Work out the finished part from the listing and answer in its coordinate system (mm). A direction names the side the tool comes from. Give positions to 0.01 mm unless a question says otherwise; leave off trailing zeros. Order: outer loops, then holes, each group sorted by start corner. A loop starts at its lowest first (then second) coordinate and runs counter-clockwise, first axis right, second up. Notation, with made-up numbers: (-33.75, 27.5) - (0.25, 27.5) arc R20 ccw to (0.25, 40.5) - close; hole circle Ø9 at (7.25, 32). An arc over 180 degrees is marked (long way). Put each result on its own line as item: value.
```python
from build123d import *

# Parameters (mm, degrees)
REVOLVE1_ANGLE      = 75
FILLET1_R           = 80
FILLET2_R           = 80
SKETCH3_W           = 220
SKETCH3_H           = 208.906104004
CUT_EXTRUDE3_DEPTH  = 159
BOSS_EXTRUDE1_START = -20
BOSS_EXTRUDE1_DEPTH = 20
SKETCH6_W           = 10
SKETCH6_H           = 10
CUT_EXTRUDE4_DEPTH  = 10


with BuildPart() as part:
    # Sketch1 → Revolve1 (revolve)
    with BuildSketch(Plane.XY):
        with BuildLine():
            Line((0, 0), (3.000014971, 0))
            Line((3.000014971, 0), (2.999985029, 0.009477573))
            add(Edge.make_bspline(
                [(2.999985029, 0.009477573), (2.993785153, 1.971956174), (2.98195041, 5.919056141), (3.145368661, 11.706950418), (3.673805689, 17.348455242), (4.826995442, 22.758009885), (6.767385374, 27.848912294), (10.462264152, 34.106073266), (16.932254921, 40.80886219), (26.377617743, 47.258644811), (36.67301066, 52.572311975), (47.441384771, 57.081049673), (62.17748954, 62.31037411), (81.042213455, 67.757539775), (104.018152235, 73.218909741), (126.982089983, 77.893970447), (142.347775171, 80.65244689), (149.958103424, 81.949720096), (150, 81.956859546)],
                knots=[0, 0, 0, 0, 0.03125, 0.0625, 0.09375, 0.125, 0.15625, 0.1875, 0.25, 0.3125, 0.375, 0.4375, 0.5, 0.625, 0.75, 0.875, 0.996633751, 0.997307001, 0.997307001, 0.997307001, 0.997307001], degree=3))
            Line((150, 81.956859546), (530, 81.956859546))
            Line((530, 81.956859546), (530, 85))
            Line((530, 85), (150, 85))
            add(Edge.make_bspline(
                [(0, 0), (-0.012294225, 3.891554312), (-0.027437579, 8.684958126), (0.361573767, 14.085722357), (0.576098453, 16.090496183), (0.782493435, 17.604822189), (0.986227589, 18.854298664), (1.188670863, 19.931536976), (1.390404268, 20.885679324), (1.591698837, 21.746529091), (1.792703864, 22.533746067), (1.993507167, 23.261083862), (2.253808552, 24.139979457), (2.580573656, 25.146175179), (2.983585386, 26.259501153), (3.385879093, 27.271261727), (3.787683439, 28.201566994), (4.189138614, 29.064817448), (4.590335615, 29.871726974), (5.05331092, 30.74778076), (5.583218589, 31.683457084), (6.185429632, 32.669732492), (6.787226927, 33.590624245), (7.451481511, 34.546094958), (8.182770444, 35.530963646), (8.985083876, 36.540013411), (9.850344603, 37.562485558), (10.782608842, 38.595746542), (11.785011743, 39.636928062), (12.851029789, 40.680352273), (13.983960321, 41.72463117), (15.186170623, 42.768194245), (16.387975322, 43.755294725), (17.654380903, 44.743506811), (18.987602276, 45.731471932), (20.389198856, 46.717890971), (21.790522044, 47.657861765), (23.257103599, 48.59836715), (24.790441056, 49.538186318), (26.391587757, 50.476245251), (28.05829275, 51.412163763), (29.791720393, 52.345056651), (31.59268286, 53.274185034), (33.459445798, 54.199628429), (35.392909821, 55.120726442), (37.459746918, 56.067201212), (39.59327023, 57.006562681), (41.860151348, 57.96659169), (44.193707143, 58.917521836), (46.660609333, 59.885320784), (49.260404933, 60.867669295), (51.99403381, 61.861671206), (54.860992187, 62.865616104), (57.794602823, 63.85555089), (60.861539281, 64.853573463), (64.06149587, 65.858380358), (67.461497598, 66.888166734), (70.995135905, 67.920234745), (74.662088876, 68.953918346), (78.462130407, 69.988575944), (82.462197069, 71.040436012), (86.662284614, 72.107100186), (91.062388571, 73.18640193), (95.662505252, 74.276388609), (100.462631288, 75.375305679), (105.462763855, 76.481579791), (110.662900527, 77.593803027), (116.063039296, 78.710717608), (121.663178505, 79.831201671), (127.529872228, 80.967142806), (133.663251007, 82.116215238), (140.063409966, 83.276352633), (145.198462089, 84.177415336), (148.333178957, 84.715838785), (149.39998937, 84.897876633), (149.733326587, 84.954653305), (149.933332963, 84.98866355), (150, 85)],
                knots=[0, 0, 0, 0, 0.061462209, 0.075705788, 0.085548437, 0.093321935, 0.099856333, 0.105553797, 0.110642995, 0.115267654, 0.119524592, 0.123482434, 0.127191759, 0.134010181, 0.140199136, 0.145901384, 0.151215493, 0.156212588, 0.160945789, 0.165455878, 0.171870938, 0.177937368, 0.183716425, 0.189254732, 0.196326298, 0.203099892, 0.209625632, 0.217492532, 0.225090541, 0.232464167, 0.24106462, 0.249438142, 0.257620809, 0.265641058, 0.274822876, 0.28384341, 0.292725747, 0.301488561, 0.311376345, 0.321146599, 0.330814589, 0.341584449, 0.352255608, 0.362840299, 0.374512001, 0.386101174, 0.398765505, 0.411352526, 0.425006218, 0.438588433, 0.453231339, 0.468927603, 0.484557057, 0.501237456, 0.517857889, 0.535527769, 0.554243231, 0.574001115, 0.593705628, 0.614453399, 0.636242373, 0.65907093, 0.682937829, 0.707842151, 0.733783254, 0.760760729, 0.78877436, 0.81782409, 0.847909993, 0.879032247, 0.912262482, 0.946527454, 0.981827786, 0.994656092, 0.99679374, 0.998931275, 1, 1, 1, 1], degree=3))
        make_face()
    revolve(axis=Axis((0, 0, 0), (1, 0, 0)), revolution_arc=REVOLVE1_ANGLE)

    # Fillet1
    fillet1_edges = [part.edges().sort_by_distance(p)[0] for p in [
        (150, 65.020748281, 49.892174934),
    ]]
    fillet(fillet1_edges, radius=FILLET1_R)

    # Fillet2
    fillet2_edges = [part.edges().sort_by_distance(p)[0] for p in [
        (150, 67.435033925, 51.744721466),
    ]]
    fillet(fillet2_edges, radius=FILLET2_R)

    # Sketch3 → Cut-Extrude3 (cut)
    with BuildSketch(Plane(origin=(0, 0, 0), x_dir=(1, 0, 0), z_dir=(0, 1, 0))):
        Rectangle(SKETCH3_W, SKETCH3_H)
    extrude(amount=CUT_EXTRUDE3_DEPTH, mode=Mode.SUBTRACT)

    # Sketch5 → Boss-Extrude1 (add)
    with BuildSketch(Plane(origin=(530, 0, 0), x_dir=(0, 0, -1), z_dir=(1, 0, 0)).offset(BOSS_EXTRUDE1_START)):
        with BuildLine():
            Line((0, 85), (0, 55))
            Line((0, 55), (-10, 55))
            Line((-10, 55), (-10, 84.409715081))
            ThreePointArc((-10, 84.409715081), (-5.008703332, 84.852300446), (0, 85))
        make_face()
    extrude(amount=BOSS_EXTRUDE1_DEPTH)

    # Sketch6 → Cut-Extrude4 (cut)
    with BuildSketch(Plane(origin=(530, 0, 0), x_dir=(0, 0, -1), z_dir=(1, 0, 0))):
        with Locations((-5, 70)):
            Rectangle(SKETCH6_W, SKETCH6_H)
    extrude(amount=-CUT_EXTRUDE4_DEPTH, mode=Mode.SUBTRACT)


solid = part.part
```
(1) Straight lines are drawn through the part: line 1 (Y direction, x = 504, z = 14); line 2 (Y direction, x = 402, z = 18.5); line 3 (Z direction, x = 157, y = 23). For each, find the intervals that lie inside material, in ascending order.
Geometry check:
line 1: y = 80.75 to 83.84
line 2: y = 79.84 to 82.96
line 3: z = 78.66 to 81.83
(2) A tool of negligible diameter and unlimited length cuts with its end or side. For faces 5 (the face through (525, 75, 5)), 6 (the face through (319.02, 21.446, 80.038)), 7 (the face through (520, 55, 5)), from which of +Z, -Z, +X, -X, +Y, -Y can it reach the whole face along a straight path? Write none if from no direction.
Geometry check:
face 5: -Z, +X
face 6: +Z, +X, -X, -Y
face 7: -Z, +X, -X, -Y
(3) Section A-A, the plane x = 324 is taken. Write down the section's boundary in (y, z).
Geometry check:
outline: (21.21, 79.16) arc R81.96 cw to (81.96, 0) - (85, 0) arc R85 ccw to (22, 82.1) - close
(4) Determine the mould class of faces 1 (the face through (110, 59, 46)), 2 (the face through (520, 70, 5)), 3 (the face through (518, 68, 10)), 4 (the face through (510, 69, 5)) for opening direction X: pulls with the +X half, pulls with the -X half, needs draft (parallel to the pull), parting line crosses it, or undercut.
Geometry check:
face 1: pulls with the -X half
face 2: pulls with the +X half
face 3: needs draft
face 4: undercut
(5) Given pin 1 (5 mm diameter, centred on y = 69.5, z = 5.5, fed in from +X); pin 2 (1 mm diameter, centred on x = 410.5, z = 16, fed in from +Y); pin 3 (1.5 mm diameter, centred on x = 457.5, z = 48, fed in from -Y), each flat-ended and moving along its own axis, determine where each tip first touches the part or whether it passes through.
Geometry check:
pin 1: stops at x = 520
pin 2: stops at y = 83.57
pin 3: stops at y = 65.88
